The model under review builds one solid part; all positions refer to its coordinate system, in mm. Face numbers are marked on the shaded views. A direction names the side the tool comes from. Give positions to 0.01 mm unless a question says otherwise; leave off trailing zeros. Order: outer loops, then holes, each group sorted by start corner. A loop starts at its lowest first (then second) coordinate and runs counter-clockwise, first axis right, second up. Notation, with made-up numbers: (54.5, 9.5) - (108.5, 9.5) arc R14 cw to (108.5, 18.5) - close; hole circle Ø11 at (23.25, -22). An arc over 180 degrees is marked (long way). Use a Markdown table: item, result. Add a question column.
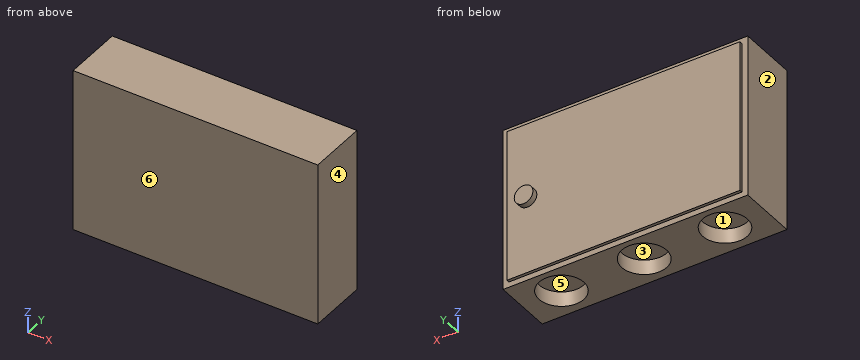
```python
from build123d import *

# Parameters (mm, degrees)
SKETCH1_W           = 248.117447686
SKETCH1_H           = 165.663783668
BOSS_EXTRUDE1_DEPTH = 60
SKETCH2_W           = 236.316367542
SKETCH2_H           = 154.827964942
BOSS_EXTRUDE2_DEPTH = 3
SKETCH3_R           = 9.48321581
BOSS_EXTRUDE3_DEPTH = 6
SKETCH4_R           = 22.698755204
SKETCH4_R_2         = 22.820518268
CUT_EXTRUDE1_DEPTH  = 15


with BuildPart() as part:
    # Sketch1 → Boss-Extrude1 (new body)
    with BuildSketch(Plane(origin=(0, 0, 0), x_dir=(1, 0, 0), z_dir=(0, 1, 0))):
        Rectangle(SKETCH1_W, SKETCH1_H)
    extrude(amount=BOSS_EXTRUDE1_DEPTH)

    # Sketch2 → Boss-Extrude2 (add)
    with BuildSketch(Plane(origin=(0, 60, 0), x_dir=(1, 0, 0), z_dir=(0, 1, 0))):
        Rectangle(SKETCH2_W, SKETCH2_H)
    extrude(amount=BOSS_EXTRUDE2_DEPTH)

    # Sketch3 → Boss-Extrude3 (add)
    with BuildSketch(Plane(origin=(0, 63, 0), x_dir=(1, 0, 0), z_dir=(0, 1, 0))):
        with Locations(Location((97.343283416, 0, 0), (0, 0, 270))):
            Circle(SKETCH3_R)
    extrude(amount=BOSS_EXTRUDE3_DEPTH)

    # Sketch4 → Cut-Extrude1 (cut)
    with BuildSketch(Plane(origin=(0, 0, -82.831891834), x_dir=(-1, 0, 0), z_dir=(0, 0, -1))):
        with Locations((-83.93255151, 31.205001036)):
            Circle(SKETCH4_R)
        with Locations((0, 31.205001036)):
            Circle(SKETCH4_R_2)
        with Locations((81.942967289, 31.205001036)):
            Circle(SKETCH4_R)
    extrude(amount=-CUT_EXTRUDE1_DEPTH, mode=Mode.SUBTRACT)


solid = part.part
```
Q1. Machinability: for the marked faces 1 and 2, which of the approach directions +Z, -Z, +X, -X, +Y, -Y give a long, thin tool a straight path to every point of the face, cutting with its end or side? Answer none if there is none.
Q2. We need section D-D (z = 0). Write out the cut boundary in (x, y), plus the area to 3 significant figures.
Q3. Draft analysis for pull direction X (two halves, no side actions). For the marked faces 3, 4, 5 and 6, state which applies: pulls with the +X half, pulls with the -X half, needs draft (parallel to the pull), parting line crosses it, or undercut.
Q4. We need section A-A (x = 46). Write out the cut boundary in (y, z).
Q5. Wall thickness on probe 1 along Y at (x, z) = (0, -79.5); probe 2 along Y at (x, z) = (0, -71); probe 3 along Y at (x, z) = (113, 2): over which ranges is each line inside the solid? List them lowest first.
Q6. We need section B-B (z = -56.5). Write out the cut boundary in (x, y).
Q7. Clearance check with flat-ended pins moving along their axes: P1, Ø13.5, axis at x = 9, y = 35, coming from the -Z side; P2, Ø0.9, axis at x = 59, y = 61, coming from the +Z side; P3, Ø1.5, axis at y = 61.5, z = -6.5, coming from the -X side; P4, Ø1.5, axis at x = -89, z = 11, coming from the -Y side. State where each tip first meets the part, or that it passes through.
Q8. We need section C-C (x = 0). Write out the cut boundary in (y, z).
Here are the results:
| question | item | result |
|---|---|---|
| 1 | face 1 | -Z |
| 1 | face 2 | +Z, -Z, -X, +Y, -Y |
| 2 | outline | (-124.06, 0) - (124.06, 0) - (124.06, 60) - (118.16, 60) - (118.16, 63) - (106.83, 63) - (106.83, 69) - (87.86, 69) - (87.86, 63) - (-118.16, 63) - (-118.16, 60) - (-124.06, 60) - close |
| 2 | area | 15,700 mm2 |
| 3 | face 3 | undercut |
| 3 | face 4 | pulls with the +X half |
| 3 | face 5 | undercut |
| 3 | face 6 | needs draft |
| 4 | outline | (0, -82.83) - (60, -82.83) - (60, -77.41) - (63, -77.41) - (63, 77.41) - (60, 77.41) - (60, 82.83) - (0, 82.83) - close |
| 5 | probe 1 | 0 to 8.38, 54.03 to 60 |
| 5 | probe 2 | 0 to 8.38, 54.03 to 63 |
| 5 | probe 3 | 0 to 63 |
| 6 | outline | (-124.06, 0) - (124.06, 0) - (124.06, 60) - (118.16, 60) - (118.16, 63) - (-118.16, 63) - (-118.16, 60) - (-124.06, 60) - close |
| 7 | P1 | z = -67.83 |
| 7 | P2 | z = 77.41 |
| 7 | P3 | x = -118.16 |
| 7 | P4 | y = 0 |
| 8 | outline | (0, -82.83) - (8.38, -82.83) - (8.38, -67.83) - (54.03, -67.83) - (54.03, -82.83) - (60, -82.83) - (60, -77.41) - (63, -77.41) - (63, 77.41) - (60, 77.41) - (60, 82.83) - (0, 82.83) - close |
